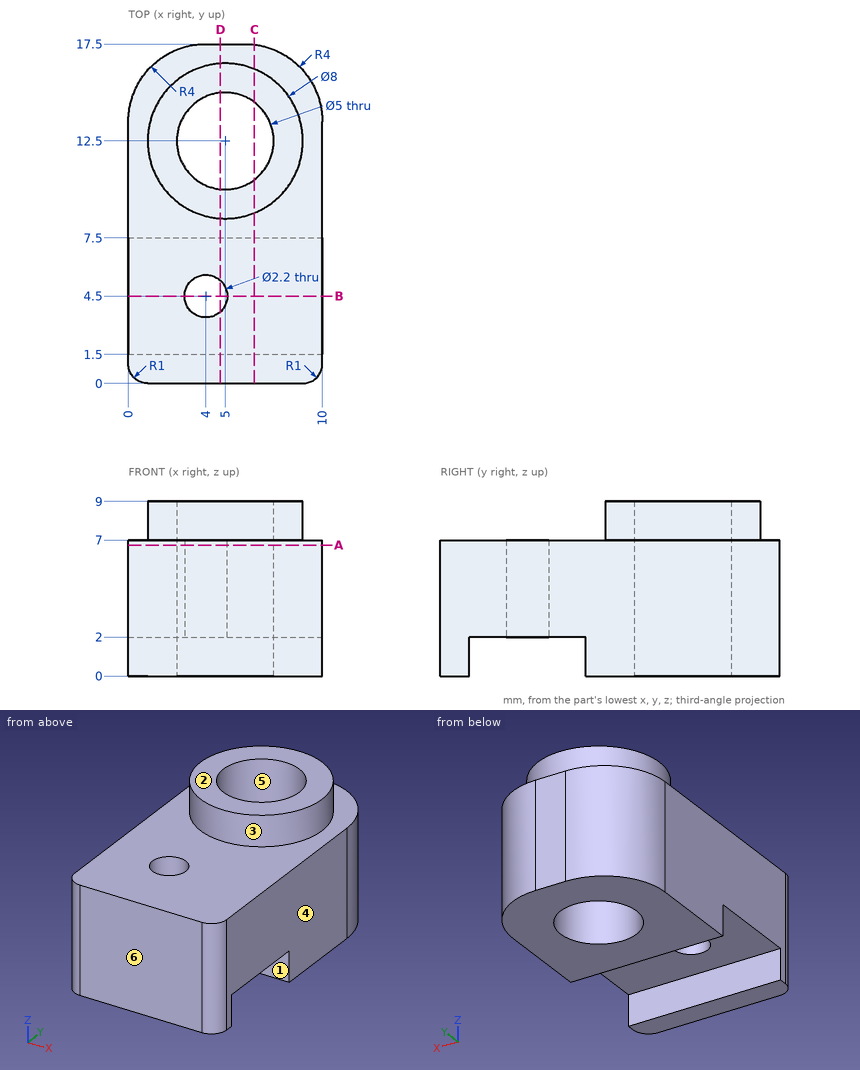
Geometry: see drawing. Coordinates: mm, zero at the bounding-box minimum. A direction names the side the tool comes from. Give positions to 0.01 mm unless a question says otherwise; leave off trailing zeros. Order: outer loops, then holes, each group sorted by start corner. A loop starts at its lowest first (then second) coordinate and runs counter-clockwise, first axis right, second up. Notation, with made-up numbers: (30, 83.5) -> (62, 83.5) arc R28 cw to (62, 119.5) -> close; hole circle Ø8 at (-24.75, -2.5). An arc over 180 degrees is marked (long way). Write item = value, one per line.
Q1. Material intervals for line 1 (Y direction, x = 5, z = 1.5); line 2 (Y direction, x = 4, z = 4.8); line 3 (X direction, y = 4.5, z = 5.6), sorted ascending. Write a range as from..to.
Data:
line_1 = 0..1.5, 7.5..10, 15..17.5
line_2 = 0..3.4, 5.6..10.21, 14.79..17.5
line_3 = 0..2.9, 5.1..10
Q2. Pin query (flat end, axial travel): pin 1 (5 mm diameter, centred on x = 2, y = 5.5, fed in from +Z); pin 2 (1.6 mm diameter, centred on x = 7.5, z = 0.5, fed in from -Y); pin 3 (3 mm diameter, centred on x = 6, y = 5, fed in from -Z). Return the tip coordinate at first contact, or that it passes through.
Data:
pin_1 = 7
pin_2 = 0
pin_3 = 2
Q3. Cut plane B-B, the plane y = 4.5. Output: boundary loops of the cut face in (x, z), and give its area (3 significant figures).
Data:
outline = (0, 2) -> (2.9, 2) -> (2.9, 7) -> (0, 7) -> close; (5.1, 2) -> (10, 2) -> (10, 7) -> (5.1, 7) -> close
area = 39.0 mm^2
Q4. Cut plane A-A, the plane z = 6.75. Output: boundary loops of the cut face in (x, y).
Data:
outline = (0, 1) arc R1 ccw to (1, 0) -> (9, 0) arc R1 ccw to (10, 1) -> (10, 13.5) arc R4 ccw to (6, 17.5) -> (4, 17.5) arc R4 ccw to (0, 13.5) -> close; hole circle Ø5 at (5, 12.5); hole circle Ø2.2 at (4, 4.5)
Q5. Set-up query: the marked faces 1, 2 and 3. Return all of +Z, -Z, +X, -X, +Y, -Y with unobstructed straight access to the full face (end or side cutting, diameter ignored); none if empty.
Data:
face_1 = -Z, +X, -X
face_2 = +Z, +X, -X, +Y, -Y
face_3 = +Z
Q6. Cut plane D-D, the plane x = 4.75. Output: boundary loops of the cut face in (y, z), and give its area (3 significant figures).
Data:
outline = (0, 0) -> (1.5, 0) -> (1.5, 2) -> (3.7, 2) -> (3.7, 7) -> (0, 7) -> close; (5.3, 2) -> (7.5, 2) -> (7.5, 0) -> (10.01, 0) -> (10.01, 9) -> (8.51, 9) -> (8.51, 7) -> (5.3, 7) -> close; (14.99, 0) -> (17.5, 0) -> (17.5, 7) -> (16.49, 7) -> (16.49, 9) -> (14.99, 9) -> close
area = 73.6 mm^2
Q7. Cut plane C-C, the plane x = 6.5. Output: boundary loops of the cut face in (y, z), and give its area (3 significant figures).
Data:
outline = (0, 0) -> (1.5, 0) -> (1.5, 2) -> (7.5, 2) -> (7.5, 0) -> (10.5, 0) -> (10.5, 9) -> (8.79, 9) -> (8.79, 7) -> (0, 7) -> close; (14.5, 0) -> (17.47, 0) -> (17.47, 7) -> (16.21, 7) -> (16.21, 9) -> (14.5, 9) -> close
area = 89.1 mm^2
Q8. Pull-direction query (X, two-part tool) for the marked faces 4, 5 and 6; classes: released by +X, released by -X, zero draft, split by the parting line, or undercut.
Data:
face_4 = released by +X
face_5 = undercut
face_6 = zero draft
